Geometry check sheet. Reference: drawing and pictorial views, mm from the part's lowest x, y, z. Round coordinates to 2 decimals unless told otherwise and drop trailing zeros. Order: outer loops, then holes, each group sorted by start corner. A loop starts at its lowest first (then second) coordinate and runs counter-clockwise, first axis right, second up.
Q1. Cross-section at B-B on x = 24. Record the cut outline in (y, z).
Q2. Cross-section at D-D on x = 3.3. Record the cut outline in (y, z).
Q3. Cross-section at C-C on y = 41.15. Record the cut outline in (x, z), then the cut area to 3 significant figures.
Q4. Cross-section at A-A on y = 30.5. Record the cut outline in (x, z) (1 decimal).
Q5. Scan lines: probe 1 along X at (y, z) = (25, 0.95) (1 decimal); probe 2 along Y at (x, z) = (79.5, 0.9); probe 3 along Y at (x, z) = (3.3, 0.7). Record each from-to range of solid material in increasing order.
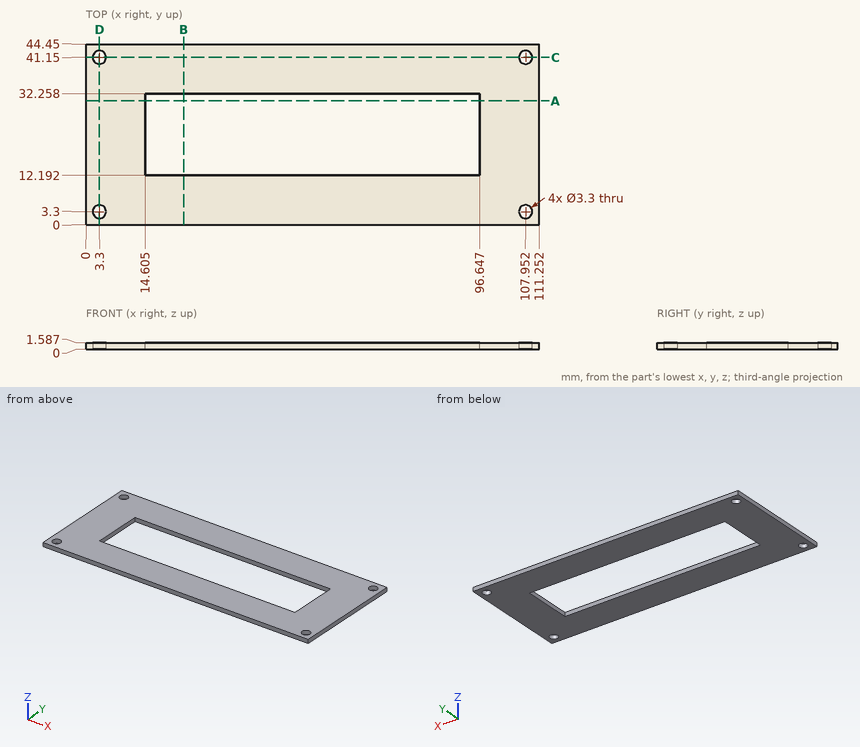
Results found:
1. outline: (0, 0) - (12.19, 0) - (12.19, 1.59) - (0, 1.59) - close; (32.26, 0) - (44.45, 0) - (44.45, 1.59) - (32.26, 1.59) - close
2. outline: (0, 0) - (1.65, 0) - (1.65, 1.59) - (0, 1.59) - close; (4.95, 0) - (39.5, 0) - (39.5, 1.59) - (4.95, 1.59) - close; (42.8, 0) - (44.45, 0) - (44.45, 1.59) - (42.8, 1.59) - close
3. outline: (0, 0) - (1.65, 0) - (1.65, 1.59) - (0, 1.59) - close; (4.95, 0) - (106.3, 0) - (106.3, 1.59) - (4.95, 1.59) - close; (109.6, 0) - (111.25, 0) - (111.25, 1.59) - (109.6, 1.59) - close
3. area: 166 mm2
4. outline: (0, 0) - (14.6, 0) - (14.6, 1.6) - (0, 1.6) - close; (96.6, 0) - (111.3, 0) - (111.3, 1.6) - (96.6, 1.6) - close
5. probe 1: x = 0 to 14.6, 96.6 to 111.3
5. probe 2: y = 0 to 12.19, 32.26 to 44.45
5. probe 3: y = 0 to 1.65, 4.95 to 39.5, 42.8 to 44.45
